Can you work these out from the model? Positions are in its coordinate system, mm. A direction names the side the tool comes from. Coordinates: 2 decimals unless noted, no trailing zeros. Order: outer loops, then holes, each group sorted by start corner. A loop starts at its lowest first (then second) coordinate and runs counter-clockwise, first axis right, second up. Notation, with made-up numbers: (63.5, 51.25) -> (74.5, 51.25) arc R36 cw to (74.5, 85.25) -> close; hole circle Ø4 at (32.25, -15). An arc over 180 degrees is marked (long way). Write item = value, one per line.
```python
from build123d import *

# Parameters (mm, degrees)
F0_R     = 12.504289
F1_DEPTH = 6
F2_R     = 1
F2_R_2   = 0.978426
F2_R_3   = 2
F4_DEPTH = 25


with BuildPart() as f1:
    # F0 (on Front) → F1 (new body)
    with BuildSketch(Plane.XZ):
        with Locations((-13.58404, 22.957029)):
            Circle(F0_R)
    extrude(amount=F1_DEPTH)


with BuildPart() as f1_1:
    # F3: moved
    add(f1.part.moved(Location((12.8, -4.5, -23.5))))

    # F2 (on Front) → F4 (join)
    with BuildSketch(Plane.XZ):
        with Locations((-2.489394, 2.438227)):
            Circle(F2_R)
        with Locations((2.351993, 2.438227)):
            Circle(F2_R_2)
        with Locations((-2.489394, -2.40316)):
            Circle(F2_R)
        with Locations((2.351993, -2.40316)):
            Circle(F2_R)
        with Locations((-0.0687, 0.017533)):
            Circle(F2_R_3)
    extrude(amount=F4_DEPTH)


solid = f1_1.part
```
Item 1: I want a section at D-D, the plane y = -9. Please give me the cut outline in (x, z), plus the area to 3 significant figures.
A:
outline = circle Ø25.01 at (-0.78, -0.54)
area = 491 mm2
Item 2: If I drill on probe 1 along X at (y, z) = (-18.5, 2.5); probe 2 along Y at (x, z) = (-3.5, -5.5); probe 3 along Z at (x, y) = (6, -5.5), over which ranges is the centre line in solid material (lowest first)?
A:
probe_1 = -3.49 to -1.49, 1.38 to 3.33
probe_2 = -10.5 to -4.5
probe_3 = -11.05 to 9.96
Item 3: I want a section at C-C, the plane z = -9. Please give me the cut outline in (x, y).
A:
outline = (-9.99, -10.5) -> (8.43, -10.5) -> (8.43, -4.5) -> (-9.99, -4.5) -> close
Item 4: I want a section at B-B, the plane x = 0.75. Please give me the cut outline in (y, z).
A:
outline = (-25, -1.81) -> (-10.5, -1.81) -> (-10.5, -12.95) -> (-4.5, -12.95) -> (-4.5, -1.81) -> (0, -1.81) -> (0, 1.84) -> (-4.5, 1.84) -> (-4.5, 11.87) -> (-10.5, 11.87) -> (-10.5, 1.84) -> (-25, 1.84) -> close
Item 5: If we mould it in two halves opening along X, with no side actions, what happens to faces 4 (the cylindrical face through (-1.536, -2.218, -2.103)), 5 (the cylindrical face through (5.94, -7.46, 10)), 6 (the flat face through (2, 0, -2))? For each: pulls with the +X half, pulls with the -X half, needs draft (parallel to the pull), parting line crosses it, or undercut.
A:
face_4 = undercut
face_5 = parting line crosses it
face_6 = needs draft
Item 6: For faces 1 (the cylindrical face through (-1.536, -17.648, -2.103)), 2 (the flat face through (2, 0, 2)), 3 (the cylindrical face through (3.306, -2.218, -2.103)), which set-ups out of +Z, -Z, +X, -X, +Y, -Y let a thin tool reach every point of the face, with its end or its side?
A:
face_1 = -Y
face_2 = +Z, -Z, +X, -X, +Y
face_3 = +Y
Item 7: I'm going to push flat-ended pins straight in: P1, Ø4, axis at x = 7, z = -1.5, coming from the -Y side; P2, Ø8, axis at x = -6, z = 8, coming from the +Y side; P3, Ø5, axis at x = -5, y = -9, coming from the +Z side. Where does each tip first touch, or does it pass through?
A:
P1 = -10.5
P2 = -4.5
P3 = 11.84
Item 8: I want a section at A-A, the plane y = -18.75. Please give me the cut outline in (x, z), plus the area to 3 significant figures.
A:
outline = circle Ø2 at (-2.49, -2.4); circle Ø2 at (-2.49, 2.44); circle Ø4 at (-0.07, 0.02); circle Ø2 at (2.35, -2.4); circle Ø1.96 at (2.35, 2.44)
area = 25.0 mm2
